The model under review builds one solid part; all positions refer to its coordinate system, in mm. A direction names the side the tool comes from. Coordinates: 2 decimals unless noted, no trailing zeros. Answer as a JSON object with one key per item and string values.
```python
from build123d import *

# Parameters (mm, degrees)
SKETCH_1_W             = 23.5
SKETCH_1_H             = 12
EXTRUDE_1_DEPTH        = 301
HOLE_WIZARD_M6_1_D     = 5
HOLE_WIZARD_M6_1_DEPTH = 15
HOLE_WIZARD_M6_1_TIP   = 1.502151548
HOLE_WIZARD_M6_2_D     = 5
HOLE_WIZARD_M6_2_DEPTH = 15
HOLE_WIZARD_M6_2_TIP   = 1.502151548
HOLE_WIZARD_M4_1_D     = 3.3
HOLE_WIZARD_M4_1_DEPTH = 10.1
HOLE_WIZARD_M4_1_TIP   = 0.991420021


with BuildPart() as part:
    # 草图1 → 凸台-拉伸1 (new, symmetric)
    with BuildSketch(Plane(origin=(0, 0, 0), x_dir=(0, 0, -1), z_dir=(1, 0, 0))):
        with BuildLine():
            Line((-14, 15), (-11.5, 15))
            Line((-11.5, 15), (-11.5, 13.5))
            Line((-11.5, 13.5), (-11.4, 13.5))
            ThreePointArc((-11.4, 13.5), (-11.117157288, 13.382842712), (-11, 13.1))
            Line((-11, 13.1), (-11, 12))
            Line((-11, 12), (-9.5, 12))
            Line((-9.5, 12), (-9.5, 15))
            Line((-9.5, 15), (-8, 15))
            Line((-8, 15), (-8, 12.5))
            Line((-8, 12.5), (-5, 12.5))
            Line((-5, 12.5), (-5, 15))
            Line((-5, 15), (5, 15))
            Line((5, 15), (5, 12.5))
            Line((5, 12.5), (8, 12.5))
            Line((8, 12.5), (8, 15))
            Line((8, 15), (9.5, 15))
            Line((9.5, 15), (9.5, 12))
            Line((9.5, 12), (11, 12))
            Line((11, 12), (11, 13.1))
            ThreePointArc((11, 13.1), (11.117157288, 13.382842712), (11.4, 13.5))
            Line((11.4, 13.5), (11.5, 13.5))
            Line((11.5, 13.5), (11.5, 15))
            Line((11.5, 15), (14, 15))
            ThreePointArc((14, 15), (14.707106781, 14.707106781), (15, 14))
            Line((15, 14), (15, 8))
            Line((15, 8), (12.5, 8))
            Line((12.5, 8), (12.5, 5))
            Line((12.5, 5), (15, 5))
            Line((15, 5), (15, -5))
            Line((15, -5), (12.5, -5))
            Line((12.5, -5), (12.5, -8))
            Line((12.5, -8), (15, -8))
            Line((15, -8), (15, -14))
            ThreePointArc((15, -14), (14.707106781, -14.707106781), (14, -15))
            Line((14, -15), (11.5, -15))
            Line((11.5, -15), (11.5, -13.5))
            Line((11.5, -13.5), (11.4, -13.5))
            ThreePointArc((11.4, -13.5), (11.117157288, -13.382842712), (11, -13.1))
            Line((11, -13.1), (11, -12))
            Line((11, -12), (9.5, -12))
            Line((9.5, -12), (9.5, -15))
            Line((9.5, -15), (8, -15))
            Line((8, -15), (8, -12.5))
            Line((8, -12.5), (5, -12.5))
            Line((5, -12.5), (5, -15))
            Line((5, -15), (-5, -15))
            Line((-5, -15), (-5, -12.5))
            Line((-5, -12.5), (-8, -12.5))
            Line((-8, -12.5), (-8, -15))
            Line((-8, -15), (-9.5, -15))
            Line((-9.5, -15), (-9.5, -12))
            Line((-9.5, -12), (-11, -12))
            Line((-11, -12), (-11, -13.1))
            ThreePointArc((-11, -13.1), (-11.117157288, -13.382842712), (-11.4, -13.5))
            Line((-11.4, -13.5), (-11.5, -13.5))
            Line((-11.5, -13.5), (-11.5, -15))
            Line((-11.5, -15), (-14, -15))
            ThreePointArc((-14, -15), (-14.707106781, -14.707106781), (-15, -14))
            Line((-15, -14), (-15, 14))
            ThreePointArc((-15, 14), (-14.707106781, 14.707106781), (-14, 15))
        make_face()
        with BuildLine():
            Line((12, -10.5), (12, -8.5))
            ThreePointArc((12, -8.5), (11.853553391, -8.146446609), (11.5, -8))
            Line((11.5, -8), (-11.5, -8))
            ThreePointArc((-11.5, -8), (-11.853553391, -8.146446609), (-12, -8.5))
            Line((-12, -8.5), (-12, -10.5))
            ThreePointArc((-12, -10.5), (-11.853553391, -10.853553391), (-11.5, -11))
            Line((-11.5, -11), (11.5, -11))
            ThreePointArc((11.5, -11), (11.853553391, -10.853553391), (12, -10.5))
        make_face(mode=Mode.SUBTRACT)
        with BuildLine():
            Line((-11.5, 11), (11.5, 11))
            ThreePointArc((11.5, 11), (11.853553391, 10.853553391), (12, 10.5))
            Line((12, 10.5), (12, 8.5))
            ThreePointArc((12, 8.5), (11.853553391, 8.146446609), (11.5, 8))
            Line((11.5, 8), (-11.5, 8))
            ThreePointArc((-11.5, 8), (-11.853553391, 8.146446609), (-12, 8.5))
            Line((-12, 8.5), (-12, 10.5))
            ThreePointArc((-12, 10.5), (-11.853553391, 10.853553391), (-11.5, 11))
        make_face(mode=Mode.SUBTRACT)
        Rectangle(SKETCH_1_W, SKETCH_1_H, mode=Mode.SUBTRACT)
    extrude(amount=EXTRUDE_1_DEPTH, both=True)

    # M6 螺纹孔1
    with Locations(Plane.XZ.offset(15)):
        with Locations((281, 0), (266, 0), (-281, 0), (-266, 0)):
            Hole(HOLE_WIZARD_M6_1_D / 2, depth=HOLE_WIZARD_M6_1_DEPTH)
            with Locations((0, 0, -(HOLE_WIZARD_M6_1_DEPTH + HOLE_WIZARD_M6_1_TIP / 2))):  # 118° drill point
                Cone(0, HOLE_WIZARD_M6_1_D / 2, HOLE_WIZARD_M6_1_TIP, mode=Mode.SUBTRACT)

    # M6 螺纹孔2
    with Locations(Plane(origin=(0, 0, -15), x_dir=(-1, 0, 0), z_dir=(0, 0, -1))):
        with Locations((-281, 0), (-266, 0), (14, 0), (29, 0), (99, 0), (114, 0)):
            Hole(HOLE_WIZARD_M6_2_D / 2, depth=HOLE_WIZARD_M6_2_DEPTH)
            with Locations((0, 0, -(HOLE_WIZARD_M6_2_DEPTH + HOLE_WIZARD_M6_2_TIP / 2))):  # 118° drill point
                Cone(0, HOLE_WIZARD_M6_2_D / 2, HOLE_WIZARD_M6_2_TIP, mode=Mode.SUBTRACT)

    # M4 螺纹孔1
    with Locations(Plane(origin=(0, 0, -15), x_dir=(-1, 0, 0), z_dir=(0, 0, -1))):
        with Locations((-226, 0), (-126, 0), (-26, 0)):
            Hole(HOLE_WIZARD_M4_1_D / 2, depth=HOLE_WIZARD_M4_1_DEPTH)
            with Locations((0, 0, -(HOLE_WIZARD_M4_1_DEPTH + HOLE_WIZARD_M4_1_TIP / 2))):  # 118° drill point
                Cone(0, HOLE_WIZARD_M4_1_D / 2, HOLE_WIZARD_M4_1_TIP, mode=Mode.SUBTRACT)


solid = part.part
```
(1) Add section A-A on x = -206. Count the separate pieces of the cut face and the enclosed holes in it, and give its area (3 significant figures).
Results list:
{"separate pieces": "1", "enclosed holes": "3", "area": "407 mm²"}
(2) For faces 4 (the face through (4, -15, 0)), 5 (the face through (4, 0, -11.75)), list the 3-axis set-ups (+Z, -Z, +X, -X, +Y, -Y) from which the entire face can be reached by the end or side of a thin tool; tool diameter is ignored.
Results list:
{"face 4": "+Z, -Z, +X, -X, -Y", "face 5": "+X, -X"}
(3) For pin 1 Ø1.5 at (y, z) = (-5, 4) entering from +X; pin 2 Ø3 at (x, y) = (281, 0) entering from -Z, all flat-tipped, find the tip position at first contact; note any pin that passes through.
Results list:
{"pin 1": "through", "pin 2": "z = 11.75"}
(4) Wall thickness on line 1 along Y through (x, z) = (-220, -9.75); line 2 along Y through (x, z) = (-180, -7.5); line 3 along Y through (x, z) = (78, -13.5): over which ranges is each line inside the solid? List them lowest first. Write a range as from..to.
Results list:
{"line 1": "-12..-11, -8..-6, 6..8, 11..12", "line 2": "-12.5..-11, -8..-6, 6..8, 11..12.5", "line 3": "-15..-8, -5..5, 8..15"}
(5) Draft analysis for pull direction Z (two halves, no side actions). For faces 1 (the face through (4, 6, 0)), 2 (the face through (4, 0, 15)), 3 (the face through (4, 0, -15)), state which applies: released by +Z, released by -Z, zero draft, split by the parting line, or undercut.
Results list:
{"face 1": "undercut", "face 2": "released by +Z", "face 3": "released by -Z"}
